Part model, mm, in its own coordinate system. A direction names the side the tool comes from. Round coordinates to 2 decimals unless told otherwise and drop trailing zeros. Write each loop counter-clockwise with the first axis right and the second up, starting at its lowest first coordinate (ties: lowest second). Pieces come first, ordered by that corner, then holes. Notation, with made-up numbers: M 74,-2 L 105,-2 A27 ccw 105,34 Z; hole C 43,35.5 d3. An arc over 180 degrees is marked long. Use a Markdown table: item, result. Add a question column.
1) Which spindle directions (+Z, -Z, +X, -X, +Y, -Y) get a long thin tool onto all of the face, cutting with end or side? Do faces 1 (the face through (-10, 3, -11)), 2 (the face through (-3, 3, 19)), 3 (the face through (3, 3, 19)), 4 (the face through (10, 3, -12)), 5 (the face through (0, 0, -2)). Say none if no direction does.
2) Slice it at D-D on y = 5.45. Write the cut outline in (x, z), plus the area to 3 significant figures.
3) Slice it at C-C on z = -27.5. Write the cut outline in (x, y), plus the area to 3 significant figures.
4) Two-plate mould, pull along Z, no slides. Class faces 6 (the face through (1.5, 2.96, -31.64)), 7 (the face through (13.079, 3.845, 16.11)), 8 (the face through (0, 3, -37.369)): released by +Z, released by -Z, zero draft, split by the parting line, or undercut.
5) Slice it at A-A on y = 3. Write the cut outline in (x, z).
6) Drop flat-ended pins along their axis: P1, Ø2, axis at x = 14, y = 3, coming from the -Z side; P2, Ø3, axis at x = 12, y = 3.5, coming from the -Z side; P3, Ø13, axis at x = 0, z = -26.87, coming from the +Y side; P4, Ø3, axis at y = 2, z = -20, coming from the -X side. Give the stop position or say it passes through.
7) Slice it at B-B on x = 14. Write the cut outline in (y, z), plus the area to 3 significant figures.
8) Wall check: probe 1 along X at (y, z) = (3, 15.85); probe 2 along Y at (x, z) = (14, 16.2); probe 3 along X at (y, z) = (4.2, -0.5). Give the ranges that are in metal, low to high.
```python
from build123d import *

# Parameters (mm, degrees)
EXTRUDE_1_DEPTH          = 6
SKETCH_3_R               = 5
CUT_EXTRUDE_1_DEPTH      = 42.909697148
CUT_EXTRUDE_3_DEPTH      = 42.909697148
CUT_EXTRUDE_3_DEPTH_BACK = 42.909697148
SKETCH_4_R               = 1.25


with BuildPart() as part:
    # 草图1 → 凸台-拉伸1 (new body)
    with BuildSketch(Plane(origin=(0, 0, 0), x_dir=(1, 0, 0), z_dir=(0, 1, 0))):
        Polygon((-10, 37.368739811), (10, 37.368739811), (10, -14.631260189), (18, -14.631260189), (18, -17.631260189), (3, -17.631260189), (3, -20.631260189), (-3, -20.631260189), (-3, -17.631260189), (-18, -17.631260189), (-18, -14.631260189), (-10, -14.631260189), align=None)
    extrude(amount=EXTRUDE_1_DEPTH)

    # 草图3 → 切除-拉伸1 (cut, through all)
    with BuildSketch(Plane.XZ):
        with Locations(Location((0, -26.868739811, 0), (0, 0, 270))):
            Circle(SKETCH_3_R)
    extrude(amount=-CUT_EXTRUDE_1_DEPTH, mode=Mode.SUBTRACT)

    # 草图4 → 切除-拉伸3 (cut, two sides: drawn at the far end of the back side and taken through both)
    with BuildSketch(Plane.XY.offset(-CUT_EXTRUDE_3_DEPTH_BACK)):
        with Locations((-14, 3)):
            Circle(SKETCH_4_R)
        with Locations((14, 3)):
            Circle(SKETCH_4_R)
    extrude(amount=CUT_EXTRUDE_3_DEPTH + CUT_EXTRUDE_3_DEPTH_BACK, mode=Mode.SUBTRACT)


solid = part.part
```
Entries:
| question | item | result |
|---|---|---|
| 1 | face 1 | -Z, -X, +Y, -Y |
| 1 | face 2 | +Z, -X, +Y, -Y |
| 1 | face 3 | +Z, +X, +Y, -Y |
| 1 | face 4 | -Z, +X, +Y, -Y |
| 1 | face 5 | +Z, -Z, +X, -X, -Y |
| 2 | outline | M -18,14.63 L -10,14.63 L -10,-37.37 L 10,-37.37 L 10,14.63 L 18,14.63 L 18,17.63 L 3,17.63 L 3,20.63 L -3,20.63 L -3,17.63 L -18,17.63 Z; hole C 0,-26.87 d10 |
| 2 | area | 1,090 mm^2 |
| 3 | outline | M -10,0 L -4.96,0 L -4.96,6 L -10,6 Z; M 4.96,0 L 10,0 L 10,6 L 4.96,6 Z |
| 3 | area | 60.5 mm^2 |
| 4 | face 6 | undercut |
| 4 | face 7 | zero draft |
| 4 | face 8 | released by -Z |
| 5 | outline | M -18,14.63 L -15.25,14.63 L -15.25,17.63 L -18,17.63 Z; M -12.75,14.63 L -10,14.63 L -10,-37.37 L 10,-37.37 L 10,14.63 L 12.75,14.63 L 12.75,17.63 L 3,17.63 L 3,20.63 L -3,20.63 L -3,17.63 L -12.75,17.63 Z; M 15.25,14.63 L 18,14.63 L 18,17.63 L 15.25,17.63 Z; hole C 0,-26.87 d10 |
| 6 | P1 | passes through |
| 6 | P2 | stops at z = 14.63 |
| 6 | P3 | stops at y = 6 |
| 6 | P4 | stops at x = -10 |
| 7 | outline | M 0,14.63 L 1.75,14.63 L 1.75,17.63 L 0,17.63 Z; M 4.25,14.63 L 6,14.63 L 6,17.63 L 4.25,17.63 Z |
| 7 | area | 10.5 mm^2 |
| 8 | probe 1 | x = -18 to -15.25, -12.75 to 12.75, 15.25 to 18 |
| 8 | probe 2 | y = 0 to 1.75, 4.25 to 6 |
| 8 | probe 3 | x = -10 to 10 |
